Verification items for the finished model (mm, model axes). Face numbers are marked on the shaded views. A direction names the side the tool comes from. Round coordinates to 2 decimals unless told otherwise and drop trailing zeros. Write each loop counter-clockwise with the first axis right and the second up, starting at its lowest first coordinate (ties: lowest second). Pieces come first, ordered by that corner, then holes. Notation, with made-up numbers: (75, 25) -> (114, 25) arc R18 ccw to (114, 58) -> close; hole circle Ø3 at (-5.5, 23.25). An arc over 180 degrees is marked (long way). Answer as a JSON object with one key per item and string values. Group by question number.
(1) Sectioned sample at A-A on x = -182.5. Record the cut outline in (y, z).
(2) Set-up check for the marked faces 1, 2 and 3: record each of +Z, -Z, +X, -X, +Y, -Y from which the full face is reachable in a straight line by a thin tool's end or side.
(3) Draft check along Z on the marked faces 4, 5 and 6. Enter one of: released by +Z, released by -Z, zero draft, split by the parting line, or undercut.
(4) Gauge pin test, flat ends, axial feed: pin 1 Ø12 at (x, z) = (-121.5, -37.5) entering from +Y; pin 2 Ø5 at (x, z) = (-138, -40) entering from -Y; pin 3 Ø18 at (x, z) = (-88.5, -1.5) entering from +Y; pin 4 Ø11 at (y, z) = (45, 0) entering from +X. Record the tip position at first contact, or that the pin passes through.
(5) Sectioned sample at D-D on z = -35. Record the cut outline in (x, y).
(6) Sectioned sample at C-C on z = 0. Record the cut outline in (x, y), and give its area (4 significant figures).
(7) Scan lines: L1, parallel to X at y = 3, z = 35; L2, parallel to Z at x = -12, y = 4; L3, parallel to Z at x = -123, y = 16.1. Record each from-to range of solid material in increasing order. Write a range as from..to.
(8) Sectioned sample at B-B on y = 45. Record the cut outline in (x, z).
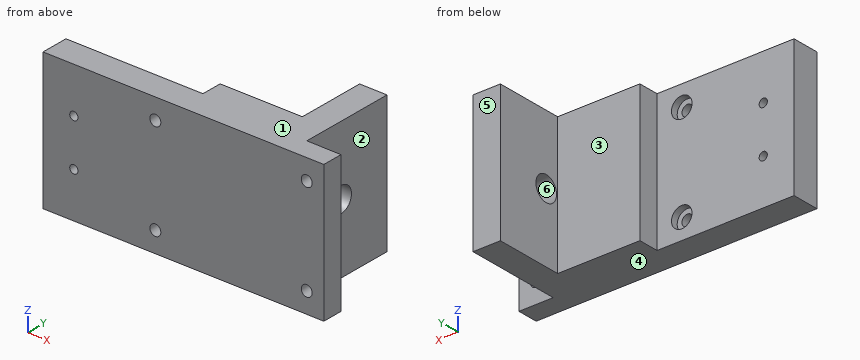
```python
from build123d import *

# Parameters (mm, degrees)
BOSS_EXTRUDE1_DEPTH = 50
SKETCH3_R           = 9
CUT_EXTRUDE1_DEPTH  = 50
SKETCH4_W           = 60
SKETCH4_H           = 42
BOSS_EXTRUDE3_DEPTH = 15
SKETCH6_R           = 3
SKETCH6_R_2         = 4
CUT_EXTRUDE3_DEPTH  = 21
SKETCH6_4_R         = 7.5
CUT_EXTRUDE4_DEPTH  = 5


with BuildPart() as part:
    # Sketch2 → Boss-Extrude1 (new body, symmetric)
    with BuildSketch(Plane.XY):
        Polygon((0, 0), (0, 15), (-25, 15), (-25, 85), (-45, 85), (-45, 35), (-105, 35), (-105, 20), (-205, 20), (-205, 0), align=None)
    extrude(amount=BOSS_EXTRUDE1_DEPTH, both=True)

    # Sketch3 → Cut-Extrude1 (cut, symmetric)
    with BuildSketch(Plane(origin=(-25, 0, 0), x_dir=(0, 0, -1), z_dir=(1, 0, 0))):
        with Locations((0, 45)):
            Circle(SKETCH3_R)
    extrude(amount=CUT_EXTRUDE1_DEPTH, both=True, mode=Mode.SUBTRACT)

    # Sketch4 → Boss-Extrude3 (add)
    with BuildSketch(Plane(origin=(0, 35, 0), x_dir=(1, 0, 0), z_dir=(0, 1, 0))):
        with Locations((-75, 0)):
            Rectangle(SKETCH4_W, SKETCH4_H)
    extrude(amount=-BOSS_EXTRUDE3_DEPTH)

    # Sketch6 → Cut-Extrude3 (cut, through all)
    with BuildSketch(Plane(origin=(0, 20, 0), x_dir=(1, 0, 0), z_dir=(0, 1, 0))):
        with Locations((-182.5, 17)):
            Circle(SKETCH6_R)
        with Locations((-123, 35)):
            Circle(SKETCH6_R_2)
        with Locations((-12.5, 35)):
            Circle(SKETCH6_R_2)
        with Locations((-12.5, -35)):
            Circle(SKETCH6_R_2)
        with Locations((-123, -35)):
            Circle(SKETCH6_R_2)
        with Locations((-182.5, -17)):
            Circle(SKETCH6_R)
    extrude(amount=-CUT_EXTRUDE3_DEPTH, mode=Mode.SUBTRACT)

    # Sketch6<4> → Cut-Extrude4 (cut)
    with BuildSketch(Plane(origin=(0, 20, 0), x_dir=(1, 0, 0), z_dir=(0, 1, 0))):
        with Locations((-123, 35)):
            Circle(SKETCH6_4_R)
        with Locations((-12.5, 35)):
            Circle(SKETCH6_4_R)
        with Locations((-12.5, -35)):
            Circle(SKETCH6_4_R)
        with Locations((-123, -35)):
            Circle(SKETCH6_4_R)
    extrude(amount=-CUT_EXTRUDE4_DEPTH, mode=Mode.SUBTRACT)


solid = part.part
```
Computed values:
{
 "1": {"outline": "(0, -50) -> (20, -50) -> (20, -20) -> (0, -20) -> close; (0, -14) -> (20, -14) -> (20, 14) -> (0, 14) -> close; (0, 20) -> (20, 20) -> (20, 50) -> (0, 50) -> close"},
 "2": {"face 1": "+Z, +X, -X, +Y, -Y", "face 2": "+Z, -Z, +X, +Y", "face 3": "+Z, -Z, -X, +Y"},
 "3": {"face 4": "released by -Z", "face 5": "zero draft", "face 6": "undercut"},
 "4": {"pin 1": "y = 20", "pin 2": "y = 0", "pin 3": "y = 35", "pin 4": "through"},
 "5": {"outline": "(-205, 0) -> (-127, 0) -> (-127, 15) -> (-130.5, 15) -> (-130.5, 20) -> (-205, 20) -> close; (-119, 0) -> (-16.5, 0) -> (-16.5, 15) -> (-25, 15) -> (-25, 85) -> (-45, 85) -> (-45, 35) -> (-105, 35) -> (-105, 20) -> (-115.5, 20) -> (-115.5, 15) -> (-119, 15) -> close; (-8.5, 0) -> (0, 0) -> (0, 15) -> (-8.5, 15) -> close"},
 "6": {"outline": "(-205, 0) -> (0, 0) -> (0, 15) -> (-25, 15) -> (-25, 36) -> (-45, 36) -> (-45, 35) -> (-105, 35) -> (-105, 20) -> (-205, 20) -> close; (-45, 54) -> (-25, 54) -> (-25, 85) -> (-45, 85) -> close", "area": "5,815 mm2"},
 "7": {"L1": "-205..-127, -119..-16.5, -8.5..0", "L2": "-50..-38.97, -31.03..31.03, 38.97..50", "L3": "-50..-42.5, -27.5..27.5, 42.5..50"},
 "8": {"outline": "(-45, -50) -> (-25, -50) -> (-25, -9) -> (-45, -9) -> close; (-45, 9) -> (-25, 9) -> (-25, 50) -> (-45, 50) -> close"}
}
